from build123d import *

# Parameters (mm, degrees)
SKETCH1_R             = 4
BOSS_EXTRUDE1_DEPTH   = 10
CHAMFER1_SIZE         = 0.15
CHAMFER1_SIZE2        = 0.259807621
CHAMFER1_PART_2_SIZE  = 0.15
CHAMFER1_PART_2_SIZE2 = 0.259807621
M3X0_5_TAPPED_HOLE1_D = 2.5


with BuildPart() as part:
    # Sketch1 → Boss-Extrude1 (new body)
    with BuildSketch(Plane(origin=(0, 0, 0), x_dir=(1, 0, 0), z_dir=(0, 1, 0))):
        Circle(SKETCH1_R)
    extrude(amount=BOSS_EXTRUDE1_DEPTH)

    # Chamfer1
    chamfer1_edges = [part.edges().sort_by_distance(p)[0] for p in [
        (-4, 0, 0),
    ]]
    chamfer1_side = [part.faces().sort_by_distance(p)[0] for p in [
        (0, 0, 0),
    ]]
    chamfer(chamfer1_edges, length=CHAMFER1_SIZE, length2=CHAMFER1_SIZE2, reference=chamfer1_side[0])

    # Chamfer1 part 2
    chamfer1_part_2_edges = [part.edges().sort_by_distance(p)[0] for p in [
        (-4, 10, 0),
    ]]
    chamfer1_part_2_side = [part.faces().sort_by_distance(p)[0] for p in [
        (-4, 5, 0),
    ]]
    chamfer(chamfer1_part_2_edges, length=CHAMFER1_PART_2_SIZE, length2=CHAMFER1_PART_2_SIZE2, reference=chamfer1_part_2_side[0])

    # M3x0.5 Tapped Hole1 (through all)
    with Locations(Plane(origin=(0, 10, 0), x_dir=(1, 0, 0), z_dir=(0, 1, 0))):
        with Locations((0, 0)):
            Hole(M3X0_5_TAPPED_HOLE1_D / 2)


solid = part.part
Read the model definition and answer for the solid it produces. Units are mm, in the model's axes. Give positions to 0.01 mm unless a question says otherwise; leave off trailing zeros. Write each loop counter-clockwise with the first axis right and the second up, starting at its lowest first coordinate (ties: lowest second). Pieces come first, ordered by that corner, then holes. Notation, with made-up numbers: (15.25, 53.5) -> (26.25, 53.5) arc R16 ccw to (26.25, 69.5) -> close; hole circle Ø8 at (85.25, 8.25). An arc over 180 degrees is marked (long way). Answer as a JSON object with one key per item and string values. Group by question number.
1) Each of these flat-tipped pins is pushed along its axis until it touches: P1, Ø1, axis at y = 2, z = 3, coming from the -X side; P2, Ø2, axis at x = 0, z = 0, coming from the +Y side; P3, Ø4, axis at x = 2.5, y = 3.5, coming from the -Z side; P4, Ø2, axis at y = 3, z = 2.5, coming from the -X side. Where does it stop, or does it pass through?
2) The mould has two halves that part along Z. Classify faces 1 (the cylindrical face through (0.27, 4.93, 1.22)), 2 (the cylindrical face through (-0.867, 4.988, 3.905)), 3 (the flat face through (0, 10, 2)): +Z half, -Z half, draft (parallel to the pull), parting line (faces both ways), or undercut.
3) Find section A-A (x = 0). Write down the section's boundary in (y, z), and give its area (3 significant figures).
4) Find section B-B (y = 5.5). Write down the section's boundary in (x, z), and give its area (3 significant figures).
5) Consider L1, parallel to Z at x = 0, y = 2.5; L2, parallel to Z at x = -0.5, y = 3.25. Determine where each line is inside the solid, lowest interval first. Write a range as from..to.
Values follow:
{
 "1": {"P1": "stops at x = -3.12", "P2": "passes through", "P3": "stops at z = -3.97", "P4": "stops at x = -3.71"},
 "2": {"face 1": "undercut", "face 2": "parting line", "face 3": "draft"},
 "3": {"outline": "(0, -3.85) -> (0.26, -4) -> (9.85, -4) -> (10, -3.74) -> (10, -1.25) -> (0, -1.25) -> close; (0, 1.25) -> (10, 1.25) -> (10, 3.74) -> (9.85, 4) -> (0.26, 4) -> (0, 3.85) -> close", "area": "54.9 mm2"},
 "4": {"outline": "circle Ø8 at (0, 0); hole circle Ø2.5 at (0, 0)", "area": "45.4 mm2"},
 "5": {"L1": "z = -4..-1.25, 1.25..4", "L2": "z = -3.97..-1.15, 1.15..3.97"}
}
